Input: dimensioned drawing with shaded views. Units: mm. Origin: part minimum x, y, z. A direction names the side the tool comes from. Round coordinates to 2 decimals unless told otherwise and drop trailing zeros. Order: outer loops, then holes, each group sorted by start corner. A loop starts at its lowest first (then second) coordinate and runs counter-clockwise, first axis right, second up.
Item 1: First-contact query: pin 1 (3 mm diameter, centred on x = 21, y = 2.5, fed in from +Z); pin 2 (3 mm diameter, centred on x = 24.5, y = 5, fed in from -Z). Flat tips, straight axial feed; report the tip coordinate or a pass-through.
Item 2: Cut plane C-C on y = 2.95. Output: boundary loops of the cut face in (x, z) (1 decimal).
Item 3: Cut plane B-B on x = 20. Output: boundary loops of the cut face in (y, z), then the cut area to 3 significant figures.
Item 4: Mould query, pull axis Z, two halves, no side actions, for the marked faces 1, 2 and 3. Classes: released by +Z, released by -Z, zero draft, split by the parting line, or undercut.
Item 5: Reachability of the marked faces 4, 5 and 6 from +Z, -Z, +X, -X, +Y, -Y: full face, straight path, thin tool, end or side. Return the list, or none.
Item 6: Cut plane A-A on z = 60.5. Output: boundary loops of the cut face in (x, y), then the cut area to 3 significant figures.
Item 7: Cut plane D-D on z = 41. Output: boundary loops of the cut face in (x, y) (1 decimal).
Item 8: Line query: L1, parallel to Z at x = 18, y = 2.25; L2, parallel to X at y = 1.7, z = 32 (1 decimal); L3, parallel to X at y = 4.45, z = 46.5 (1 decimal). Output: solid intervals per line, ascending.
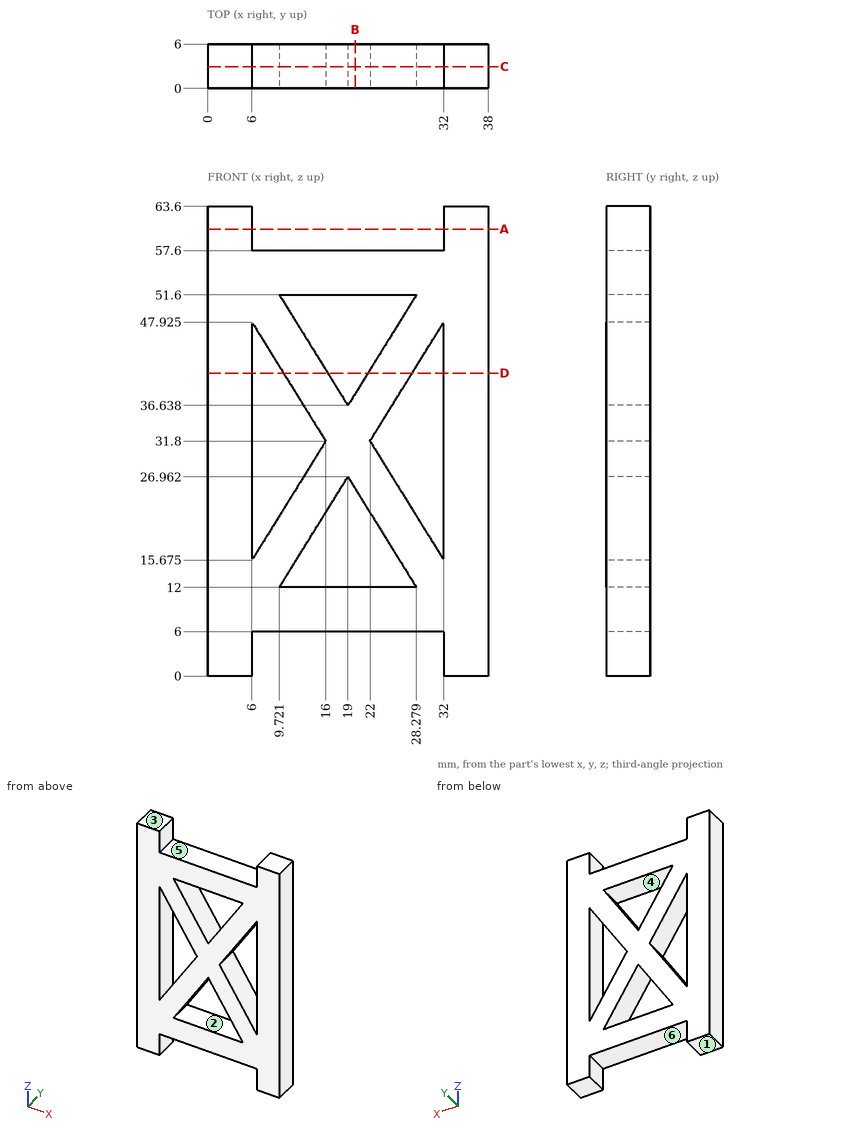
From the geometry:
1. pin 1: stops at z = 57.6
1. pin 2: stops at z = 6
2. outline: (0, 0) - (6, 0) - (6, 6) - (32, 6) - (32, 0) - (38, 0) - (38, 63.6) - (32, 63.6) - (32, 57.6) - (6, 57.6) - (6, 63.6) - (0, 63.6) - close; hole (6, 15.7) - (16, 31.8) - (6, 47.9) - close; hole (9.7, 12) - (28.3, 12) - (19, 27) - close; hole (9.7, 51.6) - (19, 36.6) - (28.3, 51.6) - close; hole (22, 31.8) - (32, 15.7) - (32, 47.9) - close
3. outline: (0, 6) - (6, 6) - (6, 12) - (0, 12) - close; (0, 25.35) - (6, 25.35) - (6, 38.25) - (0, 38.25) - close; (0, 51.6) - (6, 51.6) - (6, 57.6) - (0, 57.6) - close
3. area: 149 mm2
4. face 1: released by -Z
4. face 2: undercut
4. face 3: released by +Z
5. face 4: +Y, -Y
5. face 5: +Z, +Y, -Y
5. face 6: -Z, +Y, -Y
6. outline: (0, 0) - (6, 0) - (6, 6) - (0, 6) - close; (32, 0) - (38, 0) - (38, 6) - (32, 6) - close
6. area: 72.0 mm2
7. outline: (0, 0) - (6, 0) - (6, 6) - (0, 6) - close; (10.3, 0) - (16.3, 0) - (16.3, 6) - (10.3, 6) - close; (21.7, 0) - (27.7, 0) - (27.7, 6) - (21.7, 6) - close; (32, 0) - (38, 0) - (38, 6) - (32, 6) - close
8. L1: z = 6 to 12, 25.35 to 38.25, 51.6 to 57.6
8. L2: x = 0 to 6, 15.9 to 22.1, 32 to 38
8. L3: x = 0 to 6, 6.9 to 12.9, 25.1 to 31.1, 32 to 38
